```python
from build123d import *

# Parameters (mm, degrees)
F0_R     = 23.5
F1_DEPTH = 11.5
F2_R     = 2
F3_DEPTH = 6.2
F4_R     = 1.5
F5_DEPTH = 5
F6_SIZE2 = 3
F6_SIZE  = 10
F7_R     = 2.5
F8_R     = 9.525
F9_DEPTH = 2.032


with BuildPart() as f1:
    # F0 (on Top) → F1 (new body, symmetric)
    with BuildSketch(Plane.XY):
        Circle(F0_R)
    extrude(amount=F1_DEPTH, both=True)

    # F2 (on face) → F3 (join)
    with BuildSketch(Plane.XY.offset(11.5)):
        Circle(F2_R)
    extrude(amount=F3_DEPTH)

    # F4 (on face) → F5 (cut)
    with BuildSketch(Plane(origin=(0, 0, -11.5), x_dir=(1, 0, 0), z_dir=(0, 0, -1))):
        with Locations((0, 12.5)):
            Circle(F4_R)
        with Locations((-12.5, 0)):
            Circle(F4_R)
        with Locations((0, -12.5)):
            Circle(F4_R)
        with Locations((12.5, 0)):
            Circle(F4_R)
    extrude(amount=-F5_DEPTH, mode=Mode.SUBTRACT)

    # F6
    f6_edges = [f1.edges().sort_by_distance(p)[0] for p in [
        (-23.5, 0, 11.5),
    ]]
    f6_side = f1.faces().sort_by_distance((-22.83532, 0, 11.5))[0]
    chamfer(f6_edges, length=F6_SIZE, length2=F6_SIZE2, reference=f6_side)

    # F7
    f7_edges = [f1.edges().sort_by_distance(p)[0] for p in [
        (-23.5, 0, -11.5),
    ]]
    fillet(f7_edges, radius=F7_R)

    # F8 (on Top) → F9 (cut, symmetric)
    with BuildSketch(Plane.XY):
        Circle(F8_R)
    extrude(amount=F9_DEPTH, both=True, mode=Mode.SUBTRACT)


solid = f1.part
```
Geometry: final body of the model. Coordinates: model frame, mm. A direction names the side the tool comes from. Give positions to 0.01 mm unless a question says otherwise; leave off trailing zeros. Loops run counter-clockwise (first coordinate to the right, second up) from the corner with the lowest first, then second, coordinate; pieces in that order, holes last. Notation, with made-up numbers: (-6, 21) -> (11, 21) arc R5 cw to (11, 30) -> close; hole circle Ø6 at (28, 82). An arc over 180 degrees is marked (long way). Use CSV: the item, a comma, the result in double quotes.
(1) Cut plane D-D (z = 14.5). Output: boundary loops of the cut face in (x, y), plus the area to 3 significant figures.
From the geometry:
outline,"circle Ø4 at (0, 0)"
area,"12.6 mm^2"
(2) Access query for faces 1 (the face through (0, -2, 15)), 2 (the face through (0, 0, -2.032)), 3 (the face through (22.4, 7.1, -0.1)), 4 (the face through (11, 0, -9)), 5 (the face through (0, 0, 17.7)). Directions: +Z, -Z, +X, -X, +Y, -Y. A direction counts if a zero-diameter tool reaches every point of the face in a straight line with its end or side. Return the directions, or none.
From the geometry:
face 1,"+Z"
face 2,"none"
face 3,"+Z, -Z"
face 4,"-Z"
face 5,"+Z, +X, -X, +Y, -Y"
(3) Cut plane A-A (x = 0). Output: boundary loops of the cut face in (y, z) (3 decimals).
From the geometry:
outline,"(-23.5, -9) arc R2.5 ccw to (-21, -11.5) -> (-14, -11.5) -> (-14, -6.5) -> (-11, -6.5) -> (-11, -11.5) -> (11, -11.5) -> (11, -6.5) -> (14, -6.5) -> (14, -11.5) -> (21, -11.5) arc R2.5 ccw to (23.5, -9) -> (23.5, 8.5) -> (13.5, 11.5) -> (2, 11.5) -> (2, 17.7) -> (-2, 17.7) -> (-2, 11.5) -> (-13.5, 11.5) -> (-23.5, 8.5) -> close; hole (-9.525, -2.032) -> (9.525, -2.032) -> (9.525, 2.032) -> (-9.525, 2.032) -> close"
(4) Ray query, line 1 along Y through (x, z) = (0, 1.1) (3 decimals); line 2 along Z through (x, y) = (-1, 9); line 3 along Y through (x, z) = (6, 2). Return the intervals inside material, ascending. Write a range as [from, to].
From the geometry:
line 1,"[-23.5, -9.525], [9.525, 23.5]"
line 2,"[-11.5, -2.03], [2.03, 11.5]"
line 3,"[-22.72, -7.4], [7.4, 22.72]"
(5) Pull-direction query (Z, two-part tool) for faces 6 (the face through (0, -11, -9)), 7 (the face through (-3.062, -13.79, 11.312)), 8 (the face through (0, 0, 2.032)); classes: released by +Z, released by -Z, zero draft, split by the parting line, or undercut.
From the geometry:
face 6,"zero draft"
face 7,"released by +Z"
face 8,"undercut"
(6) Cut plane C-C (z = -7.75). Output: boundary loops of the cut face in (x, y).
From the geometry:
outline,"circle Ø47 at (0, 0); hole circle Ø3 at (-12.5, 0); hole circle Ø3 at (0, -12.5); hole circle Ø3 at (0, 12.5); hole circle Ø3 at (12.5, 0)"
(7) First-contact query: P1, Ø1.8, axis at x = 0, y = 12.5, coming from the -Z side; P2, Ø3.5, axis at x = 12.5, y = 0, coming from the +Z side; P3, Ø10, axis at y = -10.5, z = -8, coming from the +X side. Flat tips, straight axial feed; report the tip coordinate or a pass-through.
From the geometry:
P1,"z = -6.5"
P2,"z = 11.5"
P3,"x = 22.85"
